The model under review builds one solid part; all positions refer to its coordinate system, in mm. Face numbers are marked on the shaded views. A direction names the side the tool comes from. Coordinates: 2 decimals unless noted, no trailing zeros. Loops run counter-clockwise (first coordinate to the right, second up) from the corner with the lowest first, then second, coordinate; pieces in that order, holes last. Notation, with made-up numbers: (-15.75, -33.75) - (4.25, -33.75) arc R13 ccw to (4.25, -18.75) - close; hole circle Ø3 at (-7, -22). An arc over 180 degrees is marked (long way). One line per item, written item: value. Start each with the question number.
1. Mouldability with a two-part tool opening along X and no side actions: class the marked faces 1, 2 and 3 as +X half, -X half, draft (parallel to the pull), parting line (faces both ways), or undercut.
2. For the marked faces 4 and 5, list the 3-axis set-ups (+Z, -Z, +X, -X, +Y, -Y) from which the entire face can be reached by the end or side of a thin tool; tool diameter is ignored.
3. We need section A-A, the plane y = 0. Give the boundary of the cut face in (x, z).
4. To check wall thickness, follow line 1 (X direction, y = 4.5, z = 0.35); line 2 (Y direction, x = 0, z = 2.65); line 3 (Y direction, x = -1, z = 5.45). State the ranges of each line that lie inside material, in increasing order.
5. We need section C-C, the plane z = 3.95. Give the boundary of the cut face in (x, y), then the cut area to 3 significant figures.
6. We need section B-B, the plane x = 0. Give the boundary of the cut face in (y, z).
7. We need section D-D, the plane y = 5. Give the boundary of the cut face in (x, z).
8. Insertion check: P1, Ø3, axis at x = -14, z = 3.5, coming from the -Y side; P2, Ø3, axis at y = -6.5, z = 5, coming from the -X side. Each pin has a flat end and moves straight along its axis. Give the tip position at first contact, or say it passes through.
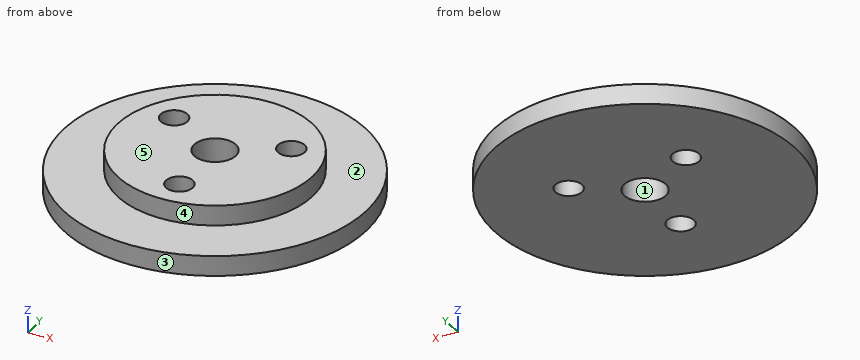
from build123d import *

# Parameters (mm, degrees)
ESQUISSE1_R             = 22.5
BOSS_EXTRU_1_DEPTH      = 3
ESQUISSE2_R             = 14.5
BOSS_EXTRU_2_DEPTH      = 3
ESQUISSE3_R             = 2
ESQUISSE3_R_2           = 3.1
ENL_V_MAT_EXTRU_1_DEPTH = 33.380549717


with BuildPart() as part:
    # Esquisse1 → Boss.-Extru.1 (new body)
    with BuildSketch(Plane.XY):
        Circle(ESQUISSE1_R)
    extrude(amount=BOSS_EXTRU_1_DEPTH)

    # Esquisse2 → Boss.-Extru.2 (add)
    with BuildSketch(Plane.XY.offset(3)):
        Circle(ESQUISSE2_R)
    extrude(amount=BOSS_EXTRU_2_DEPTH)

    # Esquisse3 → Enlèv. mat.-Extru.1 (cut, through all)
    with BuildSketch(Plane.XY.offset(6)):
        with Locations((8.660254038, 5)):
            Circle(ESQUISSE3_R)
        with Locations((-8.660254038, 5)):
            Circle(ESQUISSE3_R)
        with Locations((0, -10)):
            Circle(ESQUISSE3_R)
        Circle(ESQUISSE3_R_2)
    extrude(amount=-ENL_V_MAT_EXTRU_1_DEPTH, mode=Mode.SUBTRACT)


solid = part.part
Findings below:
1. face 1: undercut
1. face 2: draft
1. face 3: parting line
2. face 4: +Z
2. face 5: +Z, +X, -X, +Y, -Y
3. outline: (-22.5, 0) - (-3.1, 0) - (-3.1, 6) - (-14.5, 6) - (-14.5, 3) - (-22.5, 3) - close; (3.1, 0) - (22.5, 0) - (22.5, 3) - (14.5, 3) - (14.5, 6) - (3.1, 6) - close
4. line 1: -22.05 to -10.6, -6.72 to 6.72, 10.6 to 22.05
4. line 2: -22.5 to -12, -8 to -3.1, 3.1 to 22.5
4. line 3: -14.47 to -11.73, -8.27 to -2.93, 2.93 to 14.47
5. outline: circle Ø29 at (0, 0); hole circle Ø4 at (-8.66, 5); hole circle Ø6.2 at (0, 0); hole circle Ø4 at (0, -10); hole circle Ø4 at (8.66, 5)
5. area: 593 mm2
6. outline: (-22.5, 0) - (-12, 0) - (-12, 6) - (-14.5, 6) - (-14.5, 3) - (-22.5, 3) - close; (-8, 0) - (-3.1, 0) - (-3.1, 6) - (-8, 6) - close; (3.1, 0) - (22.5, 0) - (22.5, 3) - (14.5, 3) - (14.5, 6) - (3.1, 6) - close
7. outline: (-21.94, 0) - (-10.66, 0) - (-10.66, 6) - (-13.61, 6) - (-13.61, 3) - (-21.94, 3) - close; (-6.66, 0) - (6.66, 0) - (6.66, 6) - (-6.66, 6) - close; (10.66, 0) - (21.94, 0) - (21.94, 3) - (13.61, 3) - (13.61, 6) - (10.66, 6) - close
8. P1: y = -18.65
8. P2: x = -13.61
